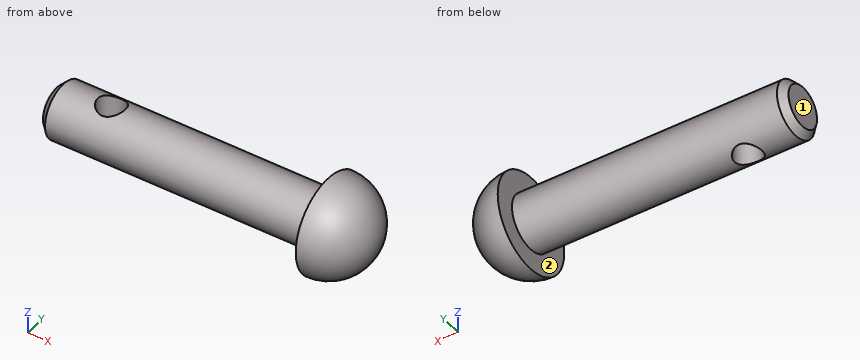
```python
from build123d import *

# Parameters (mm, degrees)
SKETCH4_R               = 1
CUT_EXTRUDE1_DEPTH      = 4.5
CUT_EXTRUDE1_DEPTH_BACK = 4.5
CHAMFER1_SIZE           = 0.5


with BuildPart() as part:
    # Sketch3 → Revolve1 (revolve)
    with BuildSketch(Plane.XY):
        with BuildLine():
            Line((-20, 0), (-20, 2))
            Line((-20, 2), (0, 2))
            Line((0, 2), (0, 3.5))
            ThreePointArc((0, 3.5), (2.474873734, 2.474873734), (3.5, 0))
            Line((3.5, 0), (-20, 0))
        make_face()
    revolve(axis=Axis((-20, 0, 0), (1, 0, 0)))

    # Sketch4 → Cut-Extrude1 (cut, two sides)
    with BuildSketch(Plane.XY) as cut_extrude1_sk:
        with Locations((-16, 0)):
            Circle(SKETCH4_R)
    extrude(amount=CUT_EXTRUDE1_DEPTH, mode=Mode.SUBTRACT)
    extrude(cut_extrude1_sk.sketch, amount=-CUT_EXTRUDE1_DEPTH_BACK, mode=Mode.SUBTRACT)

    # Chamfer1
    chamfer1_edges = [part.edges().sort_by_distance(p)[0] for p in [
        (-20, -2, 0),
    ]]
    chamfer(chamfer1_edges, length=CHAMFER1_SIZE)


solid = part.part
```
The model under review builds one solid part; all positions refer to its coordinate system, in mm. Face numbers are marked on the shaded views. A direction names the side the tool comes from. Coordinates: 2 decimals unless noted, no trailing zeros. Order: outer loops, then holes, each group sorted by start corner. A loop starts at its lowest first (then second) coordinate and runs counter-clockwise, first axis right, second up. Notation, with made-up numbers: M -3.75,82 L 46.25,82 A26 ccw 46.25,99 Z; hole C -14.75,-30 d3. An arc over 180 degrees is marked long. One line per question, with ' | ' between items.
(1) For probe 1 along X at (y, z) = (0.5, -1); probe 2 along Y at (x, z) = (-16, -1); probe 3 along X at (y, z) = (0, 0.55), list the stretches that pass through material, from the lowest coordinate up. Write a range as from..to.
Geometry results:
probe 1: x = -20..-16.87, -15.13..3.32 | probe 2: y = -1.73..-1, 1..1.73 | probe 3: x = -20..-17, -15..3.46
(2) Insertion check: pin 1 (1 mm diameter, centred on x = 0.5, z = -2.5, fed in from +Y); pin 2 (2 mm diameter, centred on y = -2.5, z = -1.5, fed in from +X); pin 3 (3 mm diameter, centred on x = -2, y = 1.5, fed in from +Z); pin 4 (1.8 mm diameter, centred on x = -16, y = 0, fed in from +Z). Each pin has a flat end and moves straight along its axis. Give the tip position at first contact, or say it passes through.
Geometry results:
pin 1: stops at y = 2.84 | pin 2: stops at x = 2.93 | pin 3: stops at z = 2 | pin 4: passes through
(3) Machinability: for the marked faces 1 and 2, which of the approach directions +Z, -Z, +X, -X, +Y, -Y give a long, thin tool a straight path to every point of the face, cutting with its end or side? Answer none if there is none.
Geometry results:
face 1: +Z, -Z, -X, +Y, -Y | face 2: -X
(4) Add section B-B, the plane x = -16. Write out the cut boundary in (y, z), then the cut area to 3 significant figures.
Geometry results:
outline: M -1,-1.73 L -1,1.73 A2 ccw Z; M 1,-1.73 A2 ccw 1,1.73 Z | area: 4.91 mm²
(5) Add section C-C, the plane x = -4. Write out the cut boundary in (y, z), then the cut area to 3 significant figures.
Geometry results:
outline: C 0,0 d4 | area: 12.6 mm²
(6) Add section D-D, the plane y = -2.5. Write out the cut boundary in (x, z), then the cut area to 3 significant figures.
Geometry results:
outline: M 0,-2.45 A2.45 ccw 0,2.45 Z | area: 9.42 mm²
(7) Add section A-A, the plane y = 0. Write out the cut boundary in (x, z).
Geometry results:
outline: M -20,-1.5 L -19.5,-2 L -17,-2 L -17,2 L -19.5,2 L -20,1.5 Z; M -15,-2 L 0,-2 L 0,-3.5 A3.5 ccw 0,3.5 L 0,2 L -15,2 Z
